from build123d import *

# Parameters (mm, degrees)
BOSS_EXTRUDE1_DEPTH            = 1.6
QQ_DEPTH                       = 7.62
BOSS_EXTRUDE3_DEPTH            = 4.1275
BOSS_EXTRUDE3_DEPTH_BACK       = 4.1275
CUT_EXTRUDE1_REACH             = 16.256
CUT_EXTRUDE1_DIRECTION_2_DEPTH = 0.508
SURFACECUT1_START              = -3.7338
SURFACECUT1_DEPTH              = 4.1656
SURFACECUT1_START_2            = 0.4318
SURFACECUT1_2_DEPTH            = 2.362
SURFACECUT1_3_OUTLINE_W        = 8.255
SURFACECUT1_3_OUTLINE_H        = 1.6
SURFACECUT1_3_DEPTH            = 2.032


# Read off the part's stored shape, not the designer's step: SurfaceCut1
with BuildPart() as part:
    # Sketch1 → Boss-Extrude1 (new body)
    with BuildSketch(Plane.XY):
        Polygon((-5.7275, -2.7938), (-5.7275, 2.7938), (5.7275, 2.7938), (5.7275, -2.7938), (5.7275, -3.7338), (-5.7275, -3.7338), align=None)
    extrude(amount=-BOSS_EXTRUDE1_DEPTH)

    # Sketch2 → qq (add)
    with BuildSketch(Plane.XY):
        Polygon((-4.6355, 1.7018), (-4.6355, 2.7938), (-5.7275, 2.7938), (-5.7275, -3.7338), (5.7275, -3.7338), (5.7275, 2.7938), (4.6355, 2.7938), (4.6355, 1.7018), (4.6355, -1.7018), (-4.6355, -1.7018), align=None)
    extrude(amount=QQ_DEPTH)

    # Sketch3 → Boss-Extrude3 (add, two sides: drawn at the far end of the back side and taken through both)
    with BuildSketch(Plane(origin=(0, 0, 0), x_dir=(0, 0, -1), z_dir=(1, 0, 0)).offset(-BOSS_EXTRUDE3_DEPTH_BACK)):
        with BuildLine():
            Line((0, 2.7938), (0, 1.9938))
            Line((0, 1.9938), (-2.54, 1.9938))
            ThreePointArc((-2.54, 1.9938), (-3.252870113, 1.853726552), (-3.859739447, 1.454334539))
            ThreePointArc((-3.859739447, 1.454334539), (-5.739869724, 0.6858), (-7.62, 1.454334539))
            Line((-7.62, 1.454334539), (-7.059609171, 2.025265461))
            ThreePointArc((-7.059609171, 2.025265461), (-5.739869724, 1.4858), (-4.420130276, 2.025265461))
            ThreePointArc((-4.420130276, 2.025265461), (-3.555570676, 2.594248239), (-2.54, 2.7938))
            Line((-2.54, 2.7938), (0, 2.7938))
        make_face()
    extrude(amount=BOSS_EXTRUDE3_DEPTH + BOSS_EXTRUDE3_DEPTH_BACK)

    # Sketch4 → Cut-Extrude1 (cut, up to next)
    with BuildSketch(Plane.ZY.offset(5.7275), mode=Mode.PRIVATE) as cut_extrude1_sk1:
        with BuildLine():
            Line((7.62, 0.6858), (7.62, 2.7938))
            Line((7.62, 2.7938), (0, 2.7938))
            Line((0, 2.7938), (0, 1.9938))
            Line((0, 1.9938), (0, 1.7398))
            Line((0, 1.7398), (2.54, 1.7398))
            ThreePointArc((2.54, 1.7398), (3.156762684, 1.618610916), (3.681815359, 1.273063971))
            ThreePointArc((3.681815359, 1.273063971), (4.628191619, 0.650236125), (5.739869724, 0.4318))
            Line((5.739869724, 0.4318), (7.62, 0.4318))
            Line((7.62, 0.4318), (7.62, 0.6858))
        make_face()
    cut_extrude1_tool1 = extrude(cut_extrude1_sk1.sketch, amount=-CUT_EXTRUDE1_REACH, mode=Mode.PRIVATE) & part.part
    cut_extrude1 = cut_extrude1_tool1.solids().sort_by_distance((-5.7275, 1.850249, 4.529461))[0]
    add(cut_extrude1, mode=Mode.SUBTRACT)

    # Sketch4 → Cut-Extrude1 direction 2 (cut)
    with BuildSketch(Plane.ZY.offset(5.7275)):
        with BuildLine():
            Line((7.62, 0.6858), (7.62, 2.7938))
            Line((7.62, 2.7938), (0, 2.7938))
            Line((0, 2.7938), (0, 1.9938))
            Line((0, 1.9938), (0, 1.7398))
            Line((0, 1.7398), (2.54, 1.7398))
            ThreePointArc((2.54, 1.7398), (3.156762684, 1.618610916), (3.681815359, 1.273063971))
            ThreePointArc((3.681815359, 1.273063971), (4.628191619, 0.650236125), (5.739869724, 0.4318))
            Line((5.739869724, 0.4318), (7.62, 0.4318))
            Line((7.62, 0.4318), (7.62, 0.6858))
        make_face()
    cut_extrude1_direction_2 = extrude(amount=CUT_EXTRUDE1_DIRECTION_2_DEPTH, mode=Mode.SUBTRACT)

    # Mirror1: Cut-Extrude1, Cut-Extrude1 direction 2 across plane
    add(cut_extrude1.mirror(Plane(origin=(0, 0, 0), x_dir=(0, 0, 1), z_dir=(1, 0, 0))), mode=Mode.SUBTRACT)
    add(cut_extrude1_direction_2.mirror(Plane(origin=(0, 0, 0), x_dir=(0, 0, 1), z_dir=(1, 0, 0))), mode=Mode.SUBTRACT)

    # SurfaceCut1 outline → SurfaceCut1 (cut)
    with BuildSketch(Plane(origin=(0, 0, 0), x_dir=(1, 0, 0), z_dir=(0, 1, 0)).offset(SURFACECUT1_START)):
        Polygon((-4.1275, 0), (-4.1275, 1.6), (-5.7275, 1.6), (-5.7275, -7.62), (5.7275, -7.62), (5.7275, 1.6), (4.1275, 1.6), (4.1275, 0), align=None)
    extrude(amount=SURFACECUT1_DEPTH, mode=Mode.SUBTRACT)

    # SurfaceCut1 2 outline → SurfaceCut1 2 (cut)
    with BuildSketch(Plane(origin=(0, 0, 0), x_dir=(1, 0, 0), z_dir=(0, 1, 0)).offset(SURFACECUT1_START_2)):
        Polygon((-4.1275, 0), (-4.1275, 1.6), (-5.7275, 1.6), (-5.7275, -7.62), (-4.6355, -7.62), (-4.6355, 0), align=None)
        Polygon((5.7275, 1.6), (4.1275, 1.6), (4.1275, 0), (4.6355, 0), (4.6355, -7.62), (5.7275, -7.62), align=None)
    extrude(amount=SURFACECUT1_2_DEPTH, mode=Mode.SUBTRACT)

    # SurfaceCut1 3 outline → SurfaceCut1 3 (cut)
    with BuildSketch(Plane(origin=(0, 0, 0), x_dir=(1, 0, 0), z_dir=(0, 1, 0)).offset(SURFACECUT1_START)):
        with Locations((0, 0.8)):
            Rectangle(SURFACECUT1_3_OUTLINE_W, SURFACECUT1_3_OUTLINE_H)
    extrude(amount=SURFACECUT1_3_DEPTH, mode=Mode.SUBTRACT)


solid = part.part
Model file for the job. Use its own axes, mm. A direction names the side the tool comes from. Give positions to 0.01 mm unless a question says otherwise; leave off trailing zeros. Write each loop counter-clockwise with the first axis right and the second up, starting at its lowest first coordinate (ties: lowest second). Pieces come first, ordered by that corner, then holes. Notation, with made-up numbers: (86, 7) - (129, 7) arc R10 ccw to (129, 21) - close; hole circle Ø11 at (61, 74). An arc over 180 degrees is marked (long way). Answer as CSV lines item,"result".
1. 3-axis set-ups, long thin cutter, end or side, ignore diameter. For faces 1 (the face through (0, 1, -1.6)), 2 (the face through (-0.06, 1.86, 3.24)): which of +Z, -Z, +X, -X, +Y, -Y reach the whole face in a straight line?
Responses:
face 1,"-Z, +X, -X, +Y, -Y"
face 2,"+X, -X, -Y"
2. Band-saw the part on D-D (z = 2.25). Write the cut outline in (x, y).
Responses:
outline,"(-4.13, 1.99) - (4.13, 1.99) - (4.13, 2.79) - (-4.13, 2.79) - close"
3. Band-saw the part on C-C (y = -0.1). Write the cut outline in (x, z).
Responses:
outline,"(-4.13, -1.6) - (4.13, -1.6) - (4.13, 0) - (-4.13, 0) - close"
4. Pin check, flat tips, straight feed: pin 1 (0.8 mm diameter, centred on x = 2, z = 1, fed in from -Y); pin 2 (3 mm diameter, centred on x = 1.5, z = 0.5, fed in from -Y). Stop position of each tip, or through.
Responses:
pin 1,"stops at y = 1.99"
pin 2,"stops at y = -1.7"
5. Two-plate mould, pull along Z, no slides. Class faces 3 (the face through (0, -1.702, -1)), 4 (the face through (-0.06, 2.59, 3.57)), 5 (the face through (-0.058, 0.686, 5.711)): +Z half, -Z half, draft (parallel to the pull), parting line (faces both ways), or undercut.
Responses:
face 3,"draft"
face 4,"+Z half"
face 5,"undercut"
6. Drill centre lines: L1, parallel to Z at x = -0.25, y = 1.8; L2, parallel to Z at x = 0, y = -1.5; L3, parallel to Y at x = 1.5, z = 1. Where is each one in solid material? Low to high. Write a range as [from, to].
Responses:
L1,"z = [-1.6, 0], [3.37, 4.7], [6.78, 7.28]"
L2,"z = [-1.6, 0]"
L3,"y = [1.99, 2.79]"
7. Band-saw the part on A-A (x = -2.5). Write the cut outline in (y, z), and give its area (3 significant figures).
Responses:
outline,"(-1.7, -1.6) - (2.79, -1.6) - (2.79, 2.54) arc R2.68 ccw to (2.03, 4.42) arc R1.88 cw to (2.03, 7.06) - (1.45, 7.62) arc R2.68 ccw to (1.45, 3.86) arc R1.88 cw to (1.99, 2.54) - (1.99, 0) - (-1.7, 0) - close"
area,"13.5 mm2"
8. Band-saw the part on B-B (y = 1.1). Write the cut outline in (x, z), and give its area (3 significant figures).
Responses:
outline,"(-4.13, -1.6) - (4.13, -1.6) - (4.13, 0) - (-4.13, 0) - close; (-4.13, 4.31) - (4.13, 4.31) - (4.13, 7.17) - (-4.13, 7.17) - close"
area,"36.9 mm2"
